Design review of the part built by this model. Coordinates are the model's own, in mm. A direction names the side the tool comes from. Coordinates: 2 decimals unless noted, no trailing zeros. Loops run counter-clockwise (first coordinate to the right, second up) from the corner with the lowest first, then second, coordinate; pieces in that order, holes last. Notation, with made-up numbers: M -22,42 L -7,42 A13 cw -7,57 Z; hole C -29.75,30.5 d10. An arc over 180 degrees is marked long. Write item = value, one per line. Start each with the question number.
Autodesk Inventor part; units mm, degrees
ref_plane "YZ Plane" through (0, 0, 0) normal (1, 0, 0) x (0, 1, 0)
ref_plane "XZ Plane" through (0, 0, 0) normal (0, 1, 0) x (-1, 0, 0)
ref_plane "XY Plane" through (0, 0, 0) normal (0, 0, 1) x (1, 0, 0)
sketch "スケッチ1" plane through (0, 0, 0) normal (0, 0, 1) x (1, 0, 0)
  circle A0 centre (0, 0) radius 19
  circle A1 centre (0, 0) radius 14
  circle A2 centre (-14, 0) radius 1.75
  circle A3 centre (0, -14) radius 1.75
  circle A4 centre (14, 0) radius 1.75
  circle A5 centre (0, 14) radius 1.75
  line L0 (-19, 0) -> (19, 0)
  dimension "d10" = 28
  dimension "d0" = 38
  dimension "d11" = 3.5
  dimension "d14" = 360
extrude "押し出し1" add sketch "スケッチ1" along normal blind 5
sketch "スケッチ2" plane through (0, 0, 5) normal (0, 0, 1) x (1, 0, 0)
  circle A0 centre (0, 0) radius 11
  line L0 (5, -9.798) -> (-5, -9.798)
  line L1 (-5, -9.798) -> (-5, 9.798)
  line L2 (-5, 9.798) -> (5, 9.798)
  line L3 (5, 9.798) -> (5, -9.798)
  line L4 (5, -9.798) -> (-5, 9.798) construction
  line L5 (-5, -9.798) -> (5, 9.798) construction
  dimension "d3" = 22
  dimension "d6" = 10
extrude "押し出し2" add sketch "スケッチ2" along normal blind 10 contours A0 L3 | L3 L0 L1 L2 | L1 A0
sketch "スケッチ3" plane through (0, 0, 0) normal (0, 0, -1) x (-1, 0, 0)
  circle A0 centre (0, 0) radius 6.15
  dimension "d7" = 12.3
extrude "押し出し3" cut sketch "スケッチ3" against normal blind 30
sketch "スケッチ4" plane through (0, 0, 0) normal (0, 0, -1) x (-1, 0, 0)
  circle A0 centre (0, 0) radius 14
  point P0 (-14, 0)
  point P1 (-9.8995, -9.8995)
  point P2 (0, -14)
  point P3 (9.8995, -9.8995)
  point P4 (14, 0)
  point P5 (9.8995, 9.8995)
  point P6 (0, 14)
  point P7 (-9.8995, 9.8995)
  dimension "d16" = 28
  dimension "d33" = 360
hole "穴1" at (9.8995, -9.8995, 0) at (9.8995, 9.8995, 0) at (-9.8995, 9.8995, 0) at (-9.8995, -9.8995, 0) direction (0, 0, 1) diameter 3.5 end through all
sketch "スケッチ5" plane through (-5, 9.798, 5) normal (0, 1, 0) x (1, 0, 0)
  line L0 (10, -10) -> (0, -10)
  line L1 (5, -10) -> (5, 0)
  line L2 (0, 0) -> (10, 0)
  point P0 (5, 5)
  point P1 (5, -5)
hole "穴2" at (0, 9.798, 10) direction (0, -1, 0) diameter 4.2 end through all
properties part number "small_tire_fixer"
Q1. Clearance check with flat-ended pins moving along their axes: P1, Ø2, axis at x = 9.9, y = -9.9, coming from the -Z side; P2, Ø5.5, axis at x = 0, z = 10, coming from the -Y side; P3, Ø3, axis at x = 7, y = -14.5, coming from the +Z side; P4, Ø4, axis at x = 14, z = 4.5, coming from the -Y side. State where each tip first meets the part, or that it passes through.
Q2. Add section C-C on z = 10. State the section outline as (x, y) points.
Q3. To check wall thickness, follow line 1 (Y direction, x = -9, z = 2.75); line 2 (Z direction, x = 0, y = 7.1); line 3 (Z direction, x = 0, y = 16). State the ranges of each line that lie inside material, in increasing order. Write a range as from..to.
Q4. Add section B-B on y = 0. State the section outline as (x, z) points, plus the area to 4 significant figures.
Q5. Add section D-D on x = 9. State the section outline as (y, z) points, plus the area to 3 significant figures.
Q6. For faces 1 (the face through (-11, 0, 10)), 2 (the face through (2.3, -9.798, 9.9)), 3 (the face through (8, -8, 5)), 4 (the face through (-2.3, 9.798, 9.9)), list the 3-axis set-ups (+Z, -Z, +X, -X, +Y, -Y) from which the entire face can be reached by the end or side of a thin tool; tool diameter is ignored.
Q7. Add section A-A on x = 0. State the section outline as (y, z) points, plus the area to 3 significant figures.
Q8. Mouldability with a two-part tool opening along X and no side actions: class faces 5 (the face through (-0.631, 7.761, 12.003)), 6 (the face through (11, 0, 10)), 7 (the face through (0, 7, 15)), 8 (the face through (-5.68, -2.36, 7.4)) as released by +X, released by -X, zero draft, split by the parting line, or undercut.
Values follow:
q1.P1 = through
q1.P2 = -9.8
q1.P3 = 5
q1.P4 = -14.73
q2.outline = M -5,-9.8 L -2.1,-9.8 L -2.1,-5.78 A6.15 cw -2.1,5.78 L -2.1,9.8 L -5,9.8 A11 ccw Z; M 2.1,-9.8 L 5,-9.8 A11 ccw 5,9.8 L 2.1,9.8 L 2.1,5.78 A6.15 cw 2.1,-5.78 Z
q3.line_1 = -16.73..-11.4, -8.4..8.4, 11.4..16.73
q3.line_2 = 0..7.9, 12.1..15
q3.line_3 = 0..5
q4.outline = M -19,0 L -6.15,0 L -6.15,15 L -11,15 L -11,5 L -19,5 Z; M 6.15,0 L 19,0 L 19,5 L 11,5 L 11,15 L 6.15,15 Z
q4.area = 225.5 mm2
q5.outline = M -16.73,0 L -11.4,0 L -11.4,5 L -16.73,5 Z; M -8.4,0 L 8.4,0 L 8.4,5 L 6.32,5 L 6.32,15 L -6.32,15 L -6.32,5 L -8.4,5 Z; M 11.4,0 L 16.73,0 L 16.73,5 L 11.4,5 Z
q5.area = 264 mm2
q6.face_1 = +Z, -X
q6.face_2 = +Z, +X, -X, -Y
q6.face_3 = +Z
q6.face_4 = +Z, +X, -X, +Y
q7.outline = M -19,0 L -6.15,0 L -6.15,7.9 L -9.8,7.9 L -9.8,5 L -19,5 Z; M -9.8,12.1 L -6.15,12.1 L -6.15,15 L -9.8,15 Z; M 6.15,0 L 19,0 L 19,5 L 9.8,5 L 9.8,7.9 L 6.15,7.9 Z; M 6.15,12.1 L 9.8,12.1 L 9.8,15 L 6.15,15 Z
q7.area = 171 mm2
q8.face_5 = undercut
q8.face_6 = released by +X
q8.face_7 = zero draft
q8.face_8 = undercut
